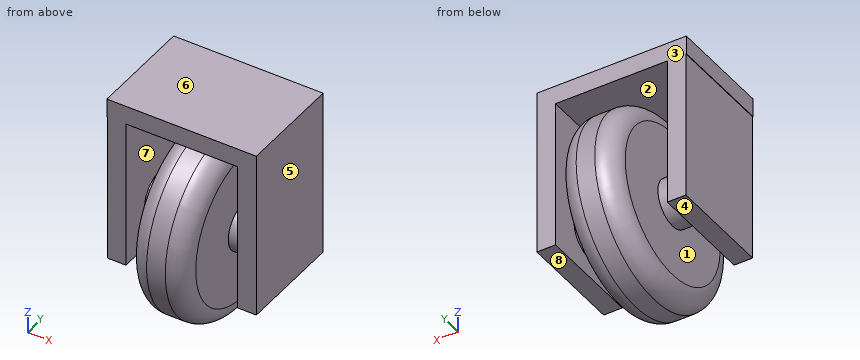
```python
from build123d import *

# Parameters (mm, degrees)
F0_R      = 127
F1_DEPTH  = 38.1
F2_R      = 31.75
F3_DEPTH  = 101.6
F4_R      = 25.4
F5_D      = 76.2
F5_DEPTH  = 12.7
F5_TIP    = 22.892789585
F6_R      = 31.75
F7_DEPTH  = 25.4
F10_DEPTH = 25.4


with BuildPart() as f1:
    # F0 (on Right) → F1 (new body, symmetric)
    with BuildSketch(Plane.YZ):
        Circle(F0_R)
    extrude(amount=F1_DEPTH, both=True)

    # F2 (on Right) → F3 (join, symmetric)
    with BuildSketch(Plane.YZ):
        Circle(F2_R)
    extrude(amount=F3_DEPTH, both=True)

    # F4
    f4_edges = [f1.edges().sort_by_distance(p)[0] for p in [
        (38.1, -127, 0),
        (-38.1, -127, 0),
    ]]
    fillet(f4_edges, radius=F4_R)

    # F5 (one way)
    with BuildSketch(Plane.YZ):
        with Locations((-0.2433381014, -0.4866788513)):
            Circle(F5_D / 2)
    extrude(amount=-F5_DEPTH, mode=Mode.SUBTRACT)
    with Locations(Plane.YZ):
        with Locations((-0.2433381014, -0.4866788513)):
            with Locations((0, 0, -(F5_DEPTH + F5_TIP / 2))):  # 118° drill point
                Cone(0, F5_D / 2, F5_TIP, mode=Mode.SUBTRACT)

    # F6 (on face) → F7 (join)
    with BuildSketch(Plane(origin=(-101.6, 0, 0), x_dir=(0, -1, 0), z_dir=(-1, 0, 0))):
        Polygon((-71.5288005566, -57.7577332966), (0, -57.7577332966), (71.5288005566, -57.7577332966), (71.5288005566, 145.4422667034), (-71.5288005566, 145.4422667034), align=None)
        Circle(F6_R, mode=Mode.SUBTRACT)
    extrude(amount=-F7_DEPTH)

    # F8: F1 across plane


with BuildPart() as f1_1:
    add(f1.part)
    add(f1.part.mirror(Plane.YZ))

    # F9 (on face) → F10 (join)
    with BuildSketch(Plane.XY.offset(145.4422667034)):
        Polygon((101.6, -71.5288005566), (101.6, 71.5288005566), (76.2, 71.5288005566), (-102.2275537252, 71.5288005566), (-102.2275537252, -71.5288005566), (76.2, -71.5288005566), align=None)
    extrude(amount=F10_DEPTH)


solid = f1_1.part
```
Can you work these out from the model? Positions are in its coordinate system, mm. Face numbers are marked on the shaded views. A direction names the side the tool comes from. Round coordinates to 2 decimals unless told otherwise and drop trailing zeros. Loops run counter-clockwise (first coordinate to the right, second up) from the corner with the lowest first, then second, coordinate; pieces in that order, holes last. Notation, with made-up numbers: M -40,30.25 L -26,30.25 A27 cw -26,69.25 Z; hole C 7,18 d11. An arc over 180 degrees is marked long. Write item = value, one per line. Start each with the question number.
(1) I need wall thicknesses on line 1 along X through (y, z) = (60, 5.5); line 2 along X through (y, z) = (-36, 130); line 3 along X through (y, z) = (60, -75). Which ranges of each line are inside material? Lowest first, please.
(2) If we mould it in two halves opening along Z, with no side actions, what happens to the marked faces 6, 7 and 8? For each: released by +Z, released by -Z, zero draft, split by the parting line, or undercut.
(3) Suppose I cut it at C-C on z = 0. Write out the boundary of the cut face in (x, y).
(4) Which directions (+Z, -Z, +X, -X, +Y, -Y) give clear straight access to the entire face, cutting with the end or side of a thin tool? Please do the marked faces 1, 2, 3, 4 and 5.
(5) Suppose I cut it at A-A on x = -46. Write out the boundary of the cut face in (y, z).
(6) Suppose I cut it at B-B on y = 0. Write out the boundary of the cut face in (x, z), plus the area to 3 significant figures.
(7) I'm going to push flat-ended pins straight in: P1, Ø2, axis at x = 26.5, z = 14.5, coming from the +Y side; P2, Ø1, axis at y = 13, z = 123, coming from the -X side; P3, Ø0.5, axis at x = -102, y = 24.5, coming from the -Z side. Where does each tip first touch, or does it pass through?
(8) Suppose I cut it at D-D on x = 89. Write out the boundary of the cut face in (y, z).
Answer block:
q1.line_1 = -101.6 to -76.2, -38.1 to 38.1, 76.2 to 101.6
q1.line_2 = -101.6 to -76.2, 76.2 to 101.6
q1.line_3 = -38.1 to 38.1
q2.face_6 = released by +Z
q2.face_7 = undercut
q2.face_8 = released by -Z
q3.outline = M -101.6,-71.53 L -76.2,-71.53 L -76.2,-31.75 L -38.1,-31.75 L -38.1,-101.6 A25.4 ccw -12.7,-127 L 12.7,-127 A25.4 ccw 38.1,-101.6 L 38.1,-31.75 L 76.2,-31.75 L 76.2,-71.53 L 101.6,-71.53 L 101.6,71.53 L 76.2,71.53 L 76.2,31.75 L 38.1,31.75 L 38.1,101.6 A25.4 ccw 12.7,127 L -12.7,127 A25.4 ccw -38.1,101.6 L -38.1,31.75 L -76.2,31.75 L -76.2,71.53 L -101.6,71.53 Z
q4.face_1 = none
q4.face_2 = +Y, -Y
q4.face_3 = +Z, +Y
q4.face_4 = -Z, -X, +Y, -Y
q4.face_5 = +Z, -Z, +X, +Y, -Y
q5.outline = M -71.53,145.44 L 71.53,145.44 L 71.53,170.84 L -71.53,170.84 Z; C 0,0 d63.5
q6.outline = M -102.23,145.44 L -101.6,145.44 L -101.6,-57.76 L -76.2,-57.76 L -76.2,-31.75 L -38.1,-31.75 L -38.1,-101.6 A25.4 ccw -12.7,-127 L 12.7,-127 A25.4 ccw 38.1,-101.6 L 38.1,-31.75 L 76.2,-31.75 L 76.2,-57.76 L 101.6,-57.76 L 101.6,170.84 L -102.23,170.84 Z; hole M -76.2,31.75 L -38.1,31.75 L -38.1,101.6 A25.4 cw -12.7,127 L 12.7,127 A25.4 cw 38.1,101.6 L 38.1,31.75 L 76.2,31.75 L 76.2,145.44 L -76.2,145.44 Z
q6.area = 39,100 mm²
q7.P1 = 122.7
q7.P2 = -101.6
q7.P3 = 145.44
q8.outline = M -71.53,-57.76 L 71.53,-57.76 L 71.53,170.84 L -71.53,170.84 Z
